```python
from build123d import *

# Parameters (mm, degrees)
BOSS_EXTRUDE1_DEPTH   = 3
SKETCH2_R             = 4
BOSS_EXTRUDE2_DEPTH   = 1.5
M5X0_8_TAPPED_HOLE1_D = 4.2
FILLET1_R             = 0.5


with BuildPart() as part:
    # Sketch1 → Boss-Extrude1 (new body)
    with BuildSketch(Plane(origin=(0, 0, 0), x_dir=(1, 0, 0), z_dir=(0, 1, 0))):
        Polygon((4.618802154, 0), (2.309401077, 4), (-2.309401077, 4), (-4.618802154, 0), (-2.309401077, -4), (2.309401077, -4), align=None)
    extrude(amount=BOSS_EXTRUDE1_DEPTH)

    # Sketch2 → Boss-Extrude2 (add)
    with BuildSketch(Plane(origin=(0, 3, 0), x_dir=(1, 0, 0), z_dir=(0, 1, 0))):
        with Locations(Location((0, 0, 0), (0, 0, 270))):
            Circle(SKETCH2_R)
    extrude(amount=BOSS_EXTRUDE2_DEPTH)

    # M5x0.8 Tapped Hole1 (through all)
    with Locations(Plane(origin=(0, 4.5, 0), x_dir=(1, 0, 0), z_dir=(0, 1, 0))):
        with Locations((0, 0)):
            Hole(M5X0_8_TAPPED_HOLE1_D / 2)

    # Fillet1
    fillet1_edges = [part.edges().sort_by_distance(p)[0] for p in [
        (0, 4.5, -4),
    ]]
    fillet(fillet1_edges, radius=FILLET1_R)


solid = part.part
```
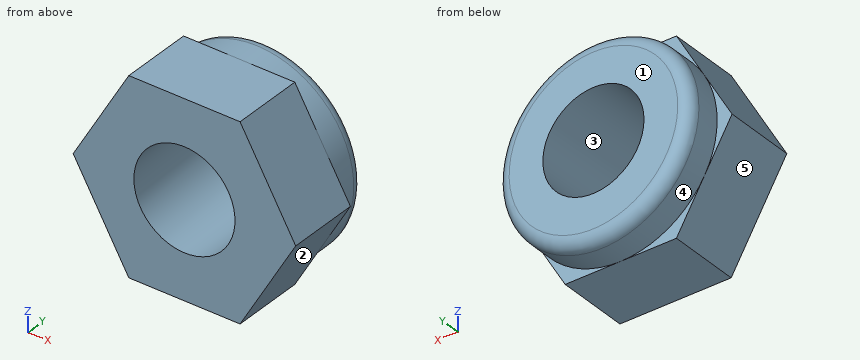
Geometry check sheet. Reference: the model listing, model coordinates, mm. Face numbers are marked on the shaded views. A direction names the side the tool comes from. Coordinates: 2 decimals unless noted, no trailing zeros. Write each loop counter-clockwise with the first axis right and the second up, starting at its lowest first coordinate (ties: lowest second). Pieces come first, ordered by that corner, then holes. Notation, with made-up numbers: M 26.25,37 L 53.25,37 A18 ccw 53.25,67 Z; hole C 84,-4.5 d4. An arc over 180 degrees is marked long. Use one line per item in the form item = value. Start each with the question number.
1) Section check B-B on y = 3.3. Enter the section's corners in (x, z), and give its area (3 significant figures).
2) Release check for a two-part mould opening along Z. For the marked faces 1, 2 and 3 record: pulls with the +Z half, pulls with the -Z half, needs draft (parallel to the pull), parting line crosses it, or undercut.
3) Set-up check for the marked faces 4 and 5: record each of +Z, -Z, +X, -X, +Y, -Y from which the full face is reachable in a straight line by a thin tool's end or side.
4) Section check A-A on y = 0.4. Enter the section's corners in (x, z), and give its area (3 significant figures).
5) Thickness scan on probe 1 along Z at (x, y) = (0, 2.2); probe 2 along X at (y, z) = (3.85, 0.25); probe 3 along X at (y, z) = (3.75, 1.5). Record the ranges inside material, lowest first. Write a range as from..to.
6) Go/stop test with flat-tipped pins: pin 1 Ø1.5 at (y, z) = (2, -1) entering from -X; pin 2 Ø3.5 at (x, z) = (0, 0) entering from -Y. Record where each tip stops, or that it passes through.
Responses:
q1.outline = C 0,0 d8; hole C 0,0 d4.2
q1.area = 36.4 mm2
q2.face_1 = needs draft
q2.face_2 = pulls with the -Z half
q2.face_3 = undercut
q3.face_4 = +Y
q3.face_5 = -Z, -X, +Y, -Y
q4.outline = M -4.62,0 L -2.31,-4 L 2.31,-4 L 4.62,0 L 2.31,4 L -2.31,4 Z; hole C 0,0 d4.2
q4.area = 41.6 mm2
q5.probe_1 = -4..-2.1, 2.1..4
q5.probe_2 = -3.99..-2.09, 2.09..3.99
q5.probe_3 = -3.71..-1.47, 1.47..3.71
q6.pin_1 = -4.47
q6.pin_2 = through
